Autodesk Inventor part; units mm, degrees
ref_plane "YZ Plane" through (0, 0, 0) normal (1, 0, 0) x (0, 1, 0)
ref_plane "XZ Plane" through (0, 0, 0) normal (0, 1, 0) x (-1, 0, 0)
ref_plane "XY Plane" through (0, 0, 0) normal (0, 0, 1) x (1, 0, 0)
sketch "Sketch1" plane through (0, 0, 0) normal (0, 1, 0) x (-1, 0, 0)
  line L0 (127.5, 90) -> (-127.5, 90)
  line L1 (-127.5, 90) -> (-127.5, -90)
  line L2 (-127.5, -90) -> (127.5, -90)
  line L3 (127.5, -90) -> (127.5, 90)
  line L4 (127.5, 90) -> (-127.5, -90) construction
  line L5 (-127.5, 90) -> (127.5, -90) construction
  point P0 (0, 0)
  dimension "d0" = 255
  dimension "d1" = 180
extrude "Extrusion1" add sketch "Sketch1" along normal blind 140
fillet "Face Fillet1" radius 20 1 edges at (127.5, 70, 90)
fillet "Face Fillet2" radius 20 1 edges at (127.5, 70, -90)
fillet "Face Fillet3" radius 20 1 edges at (-127.5, 70, -90)
fillet "Face Fillet4" radius 20 1 edges at (-127.5, 70, 90)
sketch "Sketch2" plane through (0, 140, 0) normal (0, 1, 0) x (1, 0, 0)
  line L0 (0, 0) -> (0, -90)
  line L1 (-107.5, -90) -> (107.5, -90)
  line L2 (-127.5, 70) -> (-127.5, -70)
  circle A0 centre (-90, -40.8457) radius 5
  circle A1 centre (-77.8212, -60.1893) radius 3
  dimension "d9" = 10
  dimension "d10" = 6
extrude "Extrusion2" add sketch "Sketch2" along normal blind 15
mirror "Mirror1" about plane through (0, 0, 0) normal (1, 0, 0) of "Extrusion2"
properties part number "Battery"
For this review, take the finished solid that the model builds, in its own axes (mm). A direction names the side the tool comes from. Coordinates: 2 decimals unless noted, no trailing zeros. Loops run counter-clockwise (first coordinate to the right, second up) from the corner with the lowest first, then second, coordinate; pieces in that order, holes last.
1. Insertion check: P1, Ø1, axis at x = -74.5, z = 0, coming from the +Y side. The pin has a flat end and moves straight along its axis. Give the tip position at first contact, or say it passes through.
2. Add section B-B, the plane z = -53.5. Give the boundary of the cut face in (x, y).
3. For faces 1 (the flat face through (2, 69, -90)), 2 (the cylindrical face through (80.03, 147.4, 58.16)), list the 3-axis set-ups (+Z, -Z, +X, -X, +Y, -Y) from which the entire face can be reached by the end or side of a thin tool; tool diameter is ignored.
4. Add section C-C, the plane x = 11.5. Give the boundary of the cut face in (y, z).
5. Add section A-A, the plane x = 90. Give the boundary of the cut face in (y, z), then the cut area to 4 significant figures.
6. For line 1 (Y direction, x = 8.5, z = -62.5); line 2 (X direction, y = 134.5, z = -73); line 3 (X direction, y = 12, z = 81), list the stretches that pass through material, from the lowest coordinate up.
7. Mouldability with a two-part tool opening along X and no side actions: class faces 3 (the cylindrical face through (-85.23, 147.4, 42.35)), 4 (the cylindrical face through (-80.03, 147.4, 62.22)), 5 (the flat face through (-127.5, 69, -1)), 6 (the cylindrical face through (121.486, 70.98, 84.297)) as +X half, -X half, draft (parallel to the pull), parting line (faces both ways), or undercut.
Result:
1. P1: stops at y = 140
2. outline: (-127.5, 0) - (127.5, 0) - (127.5, 140) - (-127.5, 140) - close
3. face 1: -Z, +X, -X, +Y, -Y
3. face 2: +Y
4. outline: (0, -90) - (140, -90) - (140, 90) - (0, 90) - close
5. outline: (0, -90) - (140, -90) - (140, 35.85) - (155, 35.85) - (155, 45.85) - (140, 45.85) - (140, 90) - (0, 90) - close
5. area: 25,350 mm2
6. line 1: y = 0 to 140
6. line 2: x = -127.27 to 127.27
6. line 3: x = -124.2 to 124.2
7. face 3: undercut
7. face 4: undercut
7. face 5: -X half
7. face 6: +X half
